Job drawing, mm, ordinate dimensions from the low corner. One solid piece. Round coordinates to 2 decimals unless told otherwise and drop trailing zeros. Write each loop counter-clockwise with the first axis right and the second up, starting at its lowest first coordinate (ties: lowest second). Pieces come first, ordered by that corner, then holes. Notation, with made-up numbers: (76.5, -35.5) -> (133.5, -35.5) arc R7 cw to (133.5, -25.5) -> close; hole circle Ø1 at (15, -11.5). An arc over 180 degrees is marked (long way). Use CSV: the item, a comma, the result in double quotes. Start each with the question number.
(1) Saw through at C-C (y = 11.25). Give the cut face in (x, z) (1 decimal), plus the area to 3 significant figures.
(2) Saw through at D-D (y = 2.5). Give the cut face in (x, z).
(3) Saw through at A-A (x = 5). Give the cut face in (y, z), plus the area to 3 significant figures.
(4) Drop flat-ended pins along their axis: pin 1 (4 mm diameter, centred on y = 7.5, z = 4, fed in from -X); pin 2 (5 mm diameter, centred on y = 5.5, z = 9, fed in from +X); pin 3 (1.5 mm diameter, centred on y = 17, z = 5.5, fed in from -X). Give the stop position or say it passes through.
(5) Probe line 1 (X direction, y = 11, z = 8.75); line 2 (X direction, y = 8, z = 5.5); line 3 (Y direction, x = 5, z = 5). List the from-to ranges inside material, lowest first. Write a range as [from, to].
(6) Saw through at B-B (z = 9.25). Count the separate pieces of the cut face and the enclosed holes in it, plus the area to 3 significant figures.
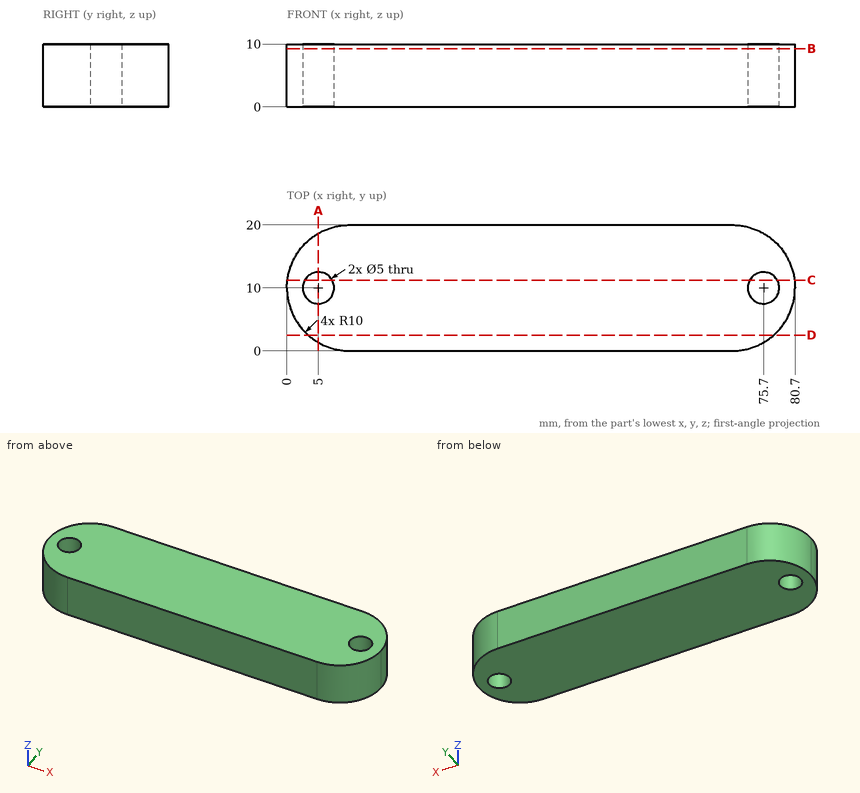
Answers:
1,outline,"(0.1, 0) -> (2.8, 0) -> (2.8, 10) -> (0.1, 10) -> close; (7.2, 0) -> (73.5, 0) -> (73.5, 10) -> (7.2, 10) -> close; (77.9, 0) -> (80.6, 0) -> (80.6, 10) -> (77.9, 10) -> close"
1,area,"719 mm²"
2,outline,"(3.39, 0) -> (77.31, 0) -> (77.31, 10) -> (3.39, 10) -> close"
3,outline,"(1.34, 0) -> (7.5, 0) -> (7.5, 10) -> (1.34, 10) -> close; (12.5, 0) -> (18.66, 0) -> (18.66, 10) -> (12.5, 10) -> close"
3,area,"123 mm²"
4,pin 1,"stops at x = 0.01"
4,pin 2,"stops at x = 80.5"
4,pin 3,"stops at x = 2.19"
5,line 1,"x = [0.05, 2.71], [7.29, 73.41], [77.99, 80.65]"
5,line 2,"x = [0.2, 3.5], [6.5, 74.2], [77.2, 80.5]"
5,line 3,"y = [1.34, 7.5], [12.5, 18.66]"
6,separate pieces,"1"
6,enclosed holes,"2"
6,area,"1,490 mm²"
